Input: part model. Units: mm. Frame: model coordinates. Face numbers are marked on the shaded views. A direction names the side the tool comes from. Round coordinates to 2 decimals unless told otherwise and drop trailing zeros. Loops run counter-clockwise (first coordinate to the right, second up) from the corner with the lowest first, then second, coordinate; pieces in that order, holes last.
(1) Line query: line 1 (Y direction, x = 37, z = -67); line 2 (Y direction, x = 18, z = -46.5); line 3 (Z direction, x = 38.5, y = -64.5). Output: solid intervals per line, ascending.
(2) Cut plane B-B, the plane x = 38. Give the number of separate pieces and of enclosed holes in the cut face, and give its area (3 significant figures).
(3) Access query for the marked faces 1, 2 and 3. Directions: +Z, -Z, +X, -X, +Y, -Y. A direction counts if a zero-diameter tool reaches every point of the face in a straight line with its end or side. Return the directions, or none.
(4) Cut plane C-C, the plane z = -38. Output: boundary loops of the cut face in (x, y), and give its area (3 significant figures).
(5) Cut plane D-D, the plane y = 45. Output: boundary loops of the cut face in (x, z), and give its area (3 significant figures).
(6) Cut plane A-A, the plane z = -68.5. Output: boundary loops of the cut face in (x, y), and give its area (3 significant figures).
(7) First-contact query: pin 1 Ø12 at (y, z) = (-102.5, -38.5) entering from -X; pin 2 Ø1.5 at (x, y) = (20, -26) entering from -Z; pin 3 Ø3 at (x, y) = (43.5, -4.5) entering from +Z; pin 4 Ø9 at (x, y) = (37, 45) entering from -Z. Flat tips, straight axial feed; report the tip coordinate or a pass-through.
(8) Draft query along Z for the marked faces 4, 5, 6 and 7. Return one class per face: released by +Z, released by -Z, zero draft, split by the parting line, or undercut.
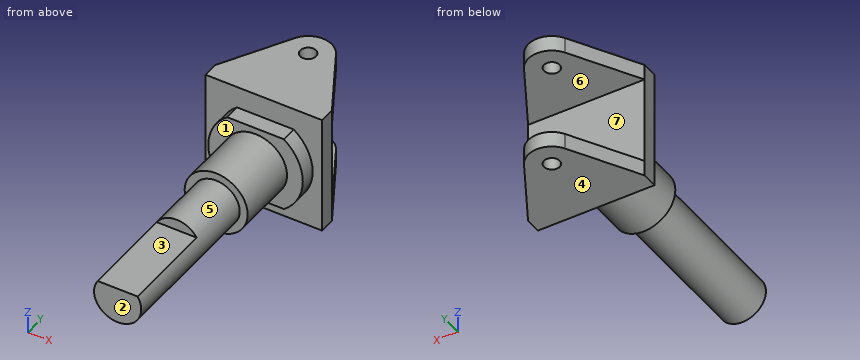
from build123d import *

# Parameters (mm, degrees)
SKETCH1_R           = 5
BOSS_EXTRUDE1_DEPTH = 76
SKETCH2_W           = 56
SKETCH2_H           = 51.048659901
CUT_EXTRUDE1_DEPTH  = 128
CUT_EXTRUDE2_START  = -10
CUT_EXTRUDE2_DEPTH  = 10
CUT_EXTRUDE3_DEPTH  = 60


with BuildPart() as part:
    # Sketch1 → Boss-Extrude1 (new body)
    with BuildSketch(Plane.XY):
        with BuildLine():
            Line((0, 0), (0, 10))
            Line((0, 10), (23.939862606, 52.377859531))
            ThreePointArc((23.939862606, 52.377859531), (36.99996154, 60), (50.06009956, 52.377926503))
            Line((50.06009956, 52.377926503), (74.000286667, 10))
            Line((74.000286667, 10), (74.000286667, 0))
            Line((74.000286667, 0), (0, 0))
        make_face()
        with Locations((37, 45)):
            Circle(SKETCH1_R, mode=Mode.SUBTRACT)
    extrude(amount=-BOSS_EXTRUDE1_DEPTH)

    # Sketch2 → Cut-Extrude1 (cut)
    with BuildSketch(Plane(origin=(0, 0, 0), x_dir=(0, 0, -1), z_dir=(1, 0, 0))):
        with Locations((38, 35.524329951)):
            Rectangle(SKETCH2_W, SKETCH2_H)
    extrude(amount=CUT_EXTRUDE1_DEPTH, mode=Mode.SUBTRACT)

    # Sketch6 → Revolve2 (revolve)
    with BuildSketch(Plane.ZY.offset(-38)):
        Polygon((-18, -10), (-8, -10), (-8, 0), (-38, 0), (-38, -150), (-23, -150), (-23, -50), (-18, -50), align=None)
    revolve(axis=Axis((38, 0, -38), (0, -1, 0)))

    # Sketch8 → Cut-Extrude2 (cut)
    with BuildSketch(Plane.XZ.offset(10).offset(CUT_EXTRUDE2_START)):
        with BuildLine():
            Line((56, -62), (20, -62))
            ThreePointArc((20, -62), (38, -68), (56, -62))
        make_face()
        with BuildLine():
            ThreePointArc((56, -14), (38, -8), (20, -14))
            Line((20, -14), (56, -14))
        make_face()
    extrude(amount=CUT_EXTRUDE2_DEPTH, mode=Mode.SUBTRACT)

    # Sketch9 → Cut-Extrude3 (cut)
    with BuildSketch(Plane.XZ.offset(150)):
        Polygon((-121.587546026, -30), (25.31142246, -30), (50.68857754, -30), (197.587546026, -30), (197.587546026, 263.79793697), (-121.587546026, 263.79793697), align=None)
    extrude(amount=-CUT_EXTRUDE3_DEPTH, mode=Mode.SUBTRACT)


solid = part.part
Reported:
1. line 1: y = 0 to 40, 50 to 60
1. line 2: y = -10 to 10
1. line 3: z = -52.99 to -23.01
2. separate pieces: 3
2. enclosed holes: 0
2. area: 6,220 mm2
3. face 1: -Y
3. face 2: +Z, -Z, +X, -X, -Y
3. face 3: +Z, +X, -X, -Y
4. outline: (0, 0) - (8, 0) - (8, -10) - (18, -10) - (18, -50) - (23, -50) - (23, -150) - (53, -150) - (53, -50) - (58, -50) - (58, -10) - (68, -10) - (68, 0) - (74, 0) - (74, 10) - (0, 10) - close
4. area: 5,940 mm2
5. outline: (19.77, -76) - (32, -76) - (32, -66) - (19.77, -66) - close; (19.77, -10) - (32, -10) - (32, 0) - (19.77, 0) - close; (42, -76) - (54.23, -76) - (54.23, -66) - (42, -66) - close; (42, -10) - (54.23, -10) - (54.23, 0) - (42, 0) - close
5. area: 489 mm2
6. outline: (0, 0) - (74, 0) - (74, 10) - (50.06, 52.38) arc R15 ccw to (23.94, 52.38) - (0, 10) - close; hole circle Ø10 at (37, 45)
6. area: 2,920 mm2
7. pin 1: stops at x = 23
7. pin 2: stops at z = -48.12
7. pin 3: stops at z = -14
7. pin 4: passes through
8. face 4: released by -Z
8. face 5: split by the parting line
8. face 6: undercut
8. face 7: undercut
